Autodesk Inventor part; units mm, degrees
ref_plane "slider_XY" through (0, 0, 0) normal (1, 0, 0) x (0, 0, -1)
ref_plane "slider_YZ" through (0, 0, 0) normal (0, 0, -1) x (0, 1, 0)
ref_plane "slider_ZX" through (0, 0, 0) normal (0, 1, 0) x (1, 0, 0)
sketch "Sketch_31" plane through (0, 0, 0) normal (1, 0, 0) x (0, 0, -1)
  line L0 (-15.5, 9) -> (-15.5, 1)
  line L1 (-15.5, 1) -> (-14.5, 0)
  line L2 (-14.5, 0) -> (14.4999, 0)
  line L3 (14.4999, 0) -> (15.5, 1)
  line L4 (15.5, 1) -> (15.5, 9)
  line L5 (15.5, 9) -> (13.15, 11.35)
  line L6 (13.15, 11.35) -> (-13.15, 11.35)
  line L7 (-13.15, 11.35) -> (-15.5, 9)
extrude "Extrusion1" add sketch "Sketch_31" along normal blind 43.6
sketch "Sketch_32" plane through (8.3, 0, 0) normal (1, 0, 0) x (0, 0, -1)
  line L0 (-16, 0.7) -> (-15.3, 0)
  line L1 (-15.3, 0) -> (15.3, 0)
  line L2 (15.3, 0) -> (16, 0.7)
  line L3 (16, 0.7) -> (16, 11.3)
  line L4 (16, 11.3) -> (15.3, 12)
  line L5 (15.3, 12) -> (8, 12)
  line L6 (8, 12) -> (7.6, 11.6)
  line L7 (7.6, 11.6) -> (-7.6, 11.6)
  line L8 (-7.6, 11.6) -> (-7.9999, 12)
  line L9 (-7.9999, 12) -> (-15.2999, 12)
  line L10 (-15.2999, 12) -> (-16, 11.3)
  line L11 (-16, 11.3) -> (-16, 0.7)
extrude "Extrusion2" add sketch "Sketch_32" along normal blind 27
sketch "Sketch_33" plane through (0, 0, 0) normal (1, 0, 0) x (0, 0, -1)
  line L0 (-7.5, 5) -> (-7.5, 4.1225)
  arc A0 (-7.25, 0.9321) -> (-7.5, 4.1225) centre (-7.5, 2.5175) ccw
  line L1 (-7.25, 0.9321) -> (-7.25, 0.25)
  line L2 (-7.25, 0.25) -> (-7.5, 0)
  line L3 (-7.5, 0) -> (-7.5, -3.5)
  line L4 (-7.5, -3.5) -> (-7, -4)
  line L5 (-7, -4) -> (6.9999, -4)
  line L6 (6.9999, -4) -> (7.5, -3.5)
  line L7 (7.5, -3.5) -> (7.5, 0)
  line L8 (7.5, 0) -> (7.25, 0.25)
  line L9 (7.25, 0.25) -> (7.25, 0.9321)
  arc A1 (7.5, 4.1225) -> (7.25, 0.9321) centre (7.5, 2.5175) ccw
  line L10 (7.5, 4.1225) -> (7.5, 5)
  line L11 (7.5, 5) -> (7, 5.5)
  line L12 (7, 5.5) -> (-7, 5.5)
  line L13 (-7, 5.5) -> (-7.5, 5)
extrude "Extrusion3" cut sketch "Sketch_33" along normal blind 43.6
sketch "Sketch4" plane through (8.3, 12, 15.2999) normal (0, 1, 0) x (1, 0, 0)
  point P0 (3.4, 2.7999)
hole "Hole1" at (11.7, 12, 12.5) direction (0, -1, 0) diameter 2.459 depth 5.2 tip angle 120 countersink diameter 3 countersink angle 90
pattern_linear "Rectangular Pattern1" count 2 spacing 20 along (1, 0, 0) count 2 spacing 25 along (0, 0, -1) of "Hole1"
sketch "Sketch_56" plane through (0, 0, 0) normal (1, 0, 0) x (0, 1, 0)
  circle A0 centre (8, 9) radius 2.49
  circle A1 centre (8, 9) radius 2.25
extrude "Extrusion4" cut sketch "Sketch_56" along normal blind 2.18
sketch "Sketch_61" plane through (0, 0, 0) normal (1, 0, 0) x (0, 1, 0)
  circle A0 centre (8, -9) radius 2.49
  circle A1 centre (8, -9) radius 2.25
extrude "Extrusion5" cut sketch "Sketch_61" along normal blind 2.18
sketch "Sketch_60" plane through (43.6, 0, 0) normal (1, 0, 0) x (0, 0, -1)
  circle A0 centre (-9, 8) radius 2.49
  circle A1 centre (-9, 8) radius 2.25
extrude "Extrusion6" cut sketch "Sketch_60" against normal blind 2.18
sketch "Sketch_63" plane through (43.6, 0, 0) normal (1, 0, 0) x (0, 0, -1)
  circle A0 centre (9, 8) radius 2.49
  circle A1 centre (9, 8) radius 2.25
extrude "Extrusion7" cut sketch "Sketch_63" against normal blind 2.18
ref_plane "slider_XY" through (0, 0, 0) normal (1, 0, 0) x (0, 0, -1)
ref_plane "slider_YZ" through (0, 0, 0) normal (0, 0, -1) x (0, 1, 0)
ref_plane "slider_ZX" through (0, 0, 0) normal (0, 1, 0) x (1, 0, 0)
properties part number "LU15ALW/O_slider_1"
Part model, mm, in its own coordinate system. A direction names the side the tool comes from. Coordinates: 2 decimals unless noted, no trailing zeros. Order: outer loops, then holes, each group sorted by start corner. A loop starts at its lowest first (then second) coordinate and runs counter-clockwise, first axis right, second up. Notation, with made-up numbers: M -4.75,52 L 50.25,52 A7 cw 50.25,63 Z; hole C 10.5,65 d11. An arc over 180 degrees is marked long. Use a Markdown table: item, result.
(1) Cut at A-A on z = -9. Write the cut outline in (x, y), then the cut area to 3 significant figures.
A:
| item | result |
|---|---|
| outline | M 0,0 L 43.6,0 L 43.6,5.51 L 41.42,5.51 L 41.42,5.75 L 43.6,5.75 L 43.6,10.25 L 41.42,10.25 L 41.42,10.49 L 43.6,10.49 L 43.6,11.35 L 35.3,11.35 L 35.3,12 L 8.3,12 L 8.3,11.35 L 0,11.35 L 0,10.49 L 2.18,10.49 L 2.18,10.25 L 0,10.25 L 0,5.75 L 2.18,5.75 L 2.18,5.51 L 0,5.51 Z |
| area | 510 mm^2 |
(2) Probe L1, parallel to X at y = 8.45, z = 12.5; L2, parallel to Z at x = 11.7, y = 10.4; L3, parallel to Y at x = 42.35, z = -9. List the from-to ranges inside material, lowest first.
A:
| item | result |
|---|---|
| L1 | x = 0 to 10.47, 12.93 to 30.47, 32.93 to 43.6 |
| L2 | z = -16 to -13.73, -11.27 to 11.27, 13.73 to 16 |
| L3 | y = 0 to 5.51, 5.75 to 10.25, 10.49 to 11.35 |
(3) Tool access for faces 4 (the cylindrical face through (12.171, 9.23, -11.364)), 5 (the flat face through (21.5, 4.6, -7.5)), 6 (the flat face through (39.4, 10.2, 14.3)), 7 (the flat face through (39, 5, -15.5)), 8 (the cylindrical face through (1.07, 6.16, -10.68)): list every direction of +Z, -Z, +X, -X, +Y, -Y with a clear straight run to the whole face (end or side of a thin tool).
A:
| item | result |
|---|---|
| face 4 | +Y |
| face 5 | +X, -X |
| face 6 | +Z, +X, +Y |
| face 7 | -Z, +X, +Y, -Y |
| face 8 | -X |
(4) Flat gauge pins, fed straight in: pin 1 (12 mm diameter, centred on x = 21, z = -1, fed in from +Y); pin 2 (4 mm diameter, centred on x = 4, y = 3, fed in from -Z); pin 3 (6.5 mm diameter, centred on x = 40.5, y = 4, fed in from +Z). Where does each tip first touch, or does it go through?
A:
| item | result |
|---|---|
| pin 1 | stops at y = 11.6 |
| pin 2 | stops at z = -15.5 |
| pin 3 | stops at z = 15.5 |
(5) Cut at C-C on z = 2. Write the cut outline in (x, y).
A:
| item | result |
|---|---|
| outline | M 0,5.5 L 43.6,5.5 L 43.6,11.35 L 35.3,11.35 L 35.3,11.6 L 8.3,11.6 L 8.3,11.35 L 0,11.35 Z |
(6) Pull direction Y, two halves, no side cores. Call faces 1 (the conical face through (31.511, 6.213, 12.599)), 2 (the cylindrical face through (32.171, 9.23, -11.364)), 3 (the cylindrical face through (21.495, 2.609, -5.898)): released by +Y, released by -Y, zero draft, split by the parting line, or undercut.
A:
| item | result |
|---|---|
| face 1 | released by +Y |
| face 2 | zero draft |
| face 3 | undercut |
(7) Cut at B-B on y = 9.5. State how many separate pieces and enclosed holes the cut face has, then the cut area to 3 significant figures.
A:
| item | result |
|---|---|
| separate pieces | 1 |
| enclosed holes | 4 |
| area | 1,340 mm^2 |
